Check sheet for the modelled part. Datum: model origin and axes. Units: mm. Face numbers are marked on the shaded views. A direction names the side the tool comes from. Round coordinates to 2 decimals unless told otherwise and drop trailing zeros. Write each loop counter-clockwise with the first axis right and the second up, starting at its lowest first coordinate (ties: lowest second). Pieces come first, ordered by that corner, then holes. Notation, with made-up numbers: (9.25, 63.5) -> (65.25, 63.5) arc R23 cw to (65.25, 93.5) -> close; hole circle Ø3 at (21.25, 85). An arc over 180 degrees is marked (long way). One line per item, written item: value.
Autodesk Inventor part; units mm, degrees
ref_plane "Work Plane3" through (0, 7.5, 0) normal (0, 1, 0) x (-1, 0, 0)
ref_plane "Work Plane4" through (0, -7.5, 0) normal (0, 1, 0) x (-1, 0, 0)
ref_plane "Work Plane5" through (-7.5, 0, 0) normal (-1, 0, 0) x (0, -1, 0)
sketch "Sketch1" plane through (0, 0, 0) normal (0, 0, 1) x (1, 0, 0)
  circle A0 centre (0, 0) radius 7.5
  dimension "d0" = 15
extrude "Extrusion1" add sketch "Sketch1" along normal blind 10 and the other way blind 28.1
sketch "Sketch2" plane through (0, 0, 10) normal (0, 0, 1) x (1, 0, 0)
  line L0 (-2.7781, -1.9844) -> (2.7781, -1.9844)
  line L1 (2.7781, -1.9844) -> (2.7781, 1.9844)
  line L2 (2.7781, 1.9844) -> (-2.7781, 1.9844)
  line L3 (-2.7781, 1.9844) -> (-2.7781, -1.9844)
  line L4 (-2.7781, -1.9844) -> (2.7781, 1.9844) construction
  line L5 (2.7781, -1.9844) -> (-2.7781, 1.9844) construction
  point P0 (0, 0)
  dimension "d3" = 5.5563
  dimension "d4" = 3.9688
extrude "Extrusion2" cut sketch "Sketch2" against normal blind 7.9375
ref_plane "Work Plane1" through (0, 0, 0) normal (0, 1, 0) x (0, 0, 1)
ref_plane "Work Plane2" through (0, 0, 0) normal (-1, 0, 0) x (0, 0, 1)
sketch "Sketch3" plane through (0, 0, 0) normal (0, 1, 0) x (0, 0, 1)
  point P0 (0, 0)
ref_plane "Work Plane3" through (0, 7.5, 0) normal (0, 1, 0) x (-1, 0, 0)
ref_plane "Work Plane4" through (0, -7.5, 0) normal (0, 1, 0) x (-1, 0, 0)
ref_plane "Work Plane5" through (-7.5, 0, 0) normal (-1, 0, 0) x (0, -1, 0)
ref_plane "Work Plane6" through (7.5, 0, 0) normal (-1, 0, 0) x (0, -1, 0)
sketch "Sketch4" plane through (0, 7.5, 0) normal (0, 1, 0) x (-1, 0, 0)
  point P0 (0, 0)
sketch "Sketch5" plane through (0, 7.5, 0) normal (0, 1, 0) x (-1, 0, 0)
  line L0 (7.5, 10) -> (-7.5, 10)
  line L1 (-2.5348, 10) -> (2.5348, 10)
  line L2 (2.5348, 10) -> (2.5348, -28.0998)
  line L3 (2.5348, -28.0998) -> (-2.5348, -28.0998)
  line L4 (-2.5348, -28.0998) -> (-2.5348, 10)
  point P0 (0, 0)
sketch "Sketch6" plane through (7.5, 0, 0) normal (-1, 0, 0) x (0, -1, 0)
  line L0 (-2.5348, 10) -> (2.5348, 10)
  line L1 (2.5348, 10) -> (2.5348, -28.0998)
  line L2 (2.5348, -28.0998) -> (-2.5348, -28.0998)
  line L3 (-2.5348, -28.0998) -> (-2.5348, 10)
  point P0 (0, 0)
sketch "Sketch7" plane through (0, -7.5, 0) normal (0, 1, 0) x (-1, 0, 0)
  point P0 (0, 0)
sketch "Sketch8" plane through (0, -7.5, 0) normal (0, 1, 0) x (-1, 0, 0)
  line L0 (-2.5348, 10) -> (2.5348, 10)
  line L1 (2.5348, 10) -> (2.5348, -28.0998)
  line L2 (2.5348, -28.0998) -> (-2.5348, -28.0998)
  line L3 (-2.5348, -28.0998) -> (-2.5348, 10)
  point P0 (0, 0)
sketch "Sketch9" plane through (0, -7.5, 0) normal (0, 1, 0) x (-1, 0, 0)
  point P0 (0, 0)
sketch "Sketch10" plane through (-7.5, 0, 0) normal (-1, 0, 0) x (0, -1, 0)
  line L0 (7.5, 10) -> (-7.5, 10)
  line L1 (-2.5422, 10) -> (2.5378, 10)
  line L2 (2.5378, 10) -> (2.5378, -28.1)
  line L3 (2.5378, -28.1) -> (-2.5422, -28.1)
  line L4 (-2.5422, -28.1) -> (-2.5422, 10)
  point P0 (0, 0)
  dimension "d9" = 5.08
  dimension "d10" = 38.1
extrude "Extrusion3" add sketch "Sketch5" along normal blind 36.83 and the other way blind 1.27
extrude "Extrusion4" add sketch "Sketch6" along normal blind 1.27 and the other way blind 36.83
extrude "Extrusion5" add sketch "Sketch10" along normal blind 36.83 and the other way blind 1.27
extrude "Extrusion6" add sketch "Sketch8" along normal blind 1.27 and the other way blind 36.83
sketch "Sketch11" plane through (0, 0, 10) normal (0, 0, 1) x (1, 0, 0)
  line L0 (2.5348, 7.0587) -> (2.5348, 6.9798)
  line L1 (44.33, 2.5348) -> (7.0587, 2.5348)
  line L2 (6.9798, 2.5348) -> (7.0587, 2.5348)
  arc A0 (2.5348, 6.9798) -> (6.9798, 2.5348) centre (6.9798, 6.9798) ccw
  arc A1 (7.0587, 2.5348) -> (2.5348, 7.0587) centre (0, 0) ccw
  arc A2 (7.0587, 2.5348) -> (2.5348, 7.0587) centre (0, 0) ccw
  arc A3 (-2.5348, 7.0587) -> (-7.0587, 2.5348) centre (0, 0) ccw
  arc A4 (-6.9798, 2.5348) -> (-2.5348, 6.9798) centre (-6.9798, 6.9798) ccw
  line L3 (-7.0587, 2.5348) -> (-6.9798, 2.5348)
  line L4 (-2.5348, 6.9798) -> (-2.5348, 7.0587)
  arc A5 (-7.0587, -2.5348) -> (-2.5348, -7.0587) centre (0, 0) ccw
  arc A6 (-2.5348, -6.9798) -> (-6.9798, -2.5348) centre (-6.9798, -6.9798) ccw
  line L5 (-2.5348, -7.0587) -> (-2.5348, -6.9798)
  line L6 (-6.9798, -2.5348) -> (-7.0587, -2.5348)
  arc A7 (2.5348, -7.0587) -> (7.0587, -2.5348) centre (0, 0) ccw
  arc A8 (6.9798, -2.5348) -> (2.5348, -6.9798) centre (6.9798, -6.9798) ccw
  line L7 (7.0587, -2.5348) -> (6.9798, -2.5348)
  line L8 (2.5348, -6.9798) -> (2.5348, -7.0587)
  dimension "d29" = 4.445
  dimension "d32" = 360
extrude "Extrusion7" cut sketch "Sketch11" against normal blind 38.1
properties part number "windmillv2"
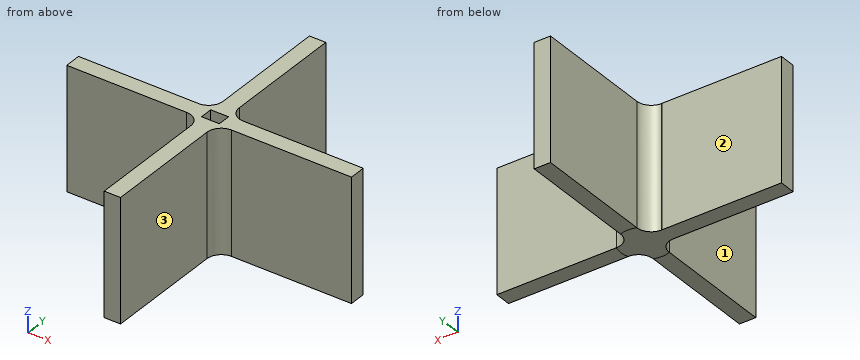
Item 1: Depth check by flat-ended pin: pin 1 (5 mm diameter, centred on x = -26, z = -6.5, fed in from +Y); pin 2 (6 mm diameter, centred on y = 31, z = 4, fed in from +X); pin 3 (10 mm diameter, centred on x = 29.5, z = -15.5, fed in from -Y). Enter the tip coordinate at first touch or a pass-through.
Result set:
pin 1: y = 2.54
pin 2: x = 2.53
pin 3: y = -2.53
Item 2: Tool access check on the marked faces 1, 2 and 3. Record the directions out of +Z, -Z, +X, -X, +Y, -Y that give a thin tool (end or side, any length) a straight path to the whole face; none if there is none.
Result set:
face 1: +Z, -Z, -X, -Y
face 2: +Z, -Z, -X, +Y
face 3: +Z, -Z, +X, -Y
Item 3: Material ranges on line 1 along X through (y, z) = (-21, -16.5); line 2 along X through (y, z) = (-3.5, -16.5), recorded low to high.
Result set:
line 1: -2.53 to 2.53
line 2: -4.21 to 4.21
Item 4: Sectioned sample at C-C (y = 15.5). Enter the section's corners in (x, z).
Result set:
outline: (-2.53, -28.1) -> (2.53, -28.1) -> (2.53, 10) -> (-2.53, 10) -> close
Item 5: Sectioned sample at B-B (x = -15). Enter the section's corners in (y, z), then the cut area to 3 significant figures.
Result set:
outline: (-2.54, -28.1) -> (2.54, -28.1) -> (2.54, 10) -> (-2.54, 10) -> close
area: 194 mm^2
